The model under review builds one solid part; all positions refer to its coordinate system, in mm. A direction names the side the tool comes from. Round coordinates to 2 decimals unless told otherwise and drop trailing zeros. Loops run counter-clockwise (first coordinate to the right, second up) from the corner with the lowest first, then second, coordinate; pieces in that order, holes last. Notation, with made-up numbers: (-38.5, 59) -> (6.5, 59) arc R20 cw to (6.5, 67) -> close; hole circle Ø9 at (78, -21). An arc over 180 degrees is marked (long way). Use a Markdown table: item, result. Add a question column.
1) Consider section B-B on y = 21.5. Give the boundary of the cut face in (x, z).
2) Consider section C-C on x = -10.5. Give the boundary of the cut face in (y, z).
3) For faces 1 (the flat face through (53.4, 3, -40.1)), 2 (the flat face through (-32.5, 23, -55)), 3 (the flat face through (41, 34, 25)), list the 3-axis set-ups (+Z, -Z, +X, -X, +Y, -Y) from which the entire face can be reached by the end or side of a thin tool; tool diameter is ignored.
4) Consider section D-D on z = -21. Give the boundary of the cut face in (x, y), plus the area to 3 significant figures.
5) Consider section A-A on z = 8.5. State how many separate pieces and enclosed holes the cut face has, plus the area to 3 significant figures.
6) Mouldability with a two-part tool opening along X and no side actions: class faces 4 (the flat face through (38, 38, 53)), 5 (the flat face through (14.5, 5, 2)), 6 (the cylindrical face through (-55.094, 1.479, 32.281)), 7 (the flat face through (-1, 0, -1)) as released by +X, released by -X, zero draft, split by the parting line, or undercut.
7) Insertion check: pin 1 (2.5 mm diameter, centred on x = 18, z = 42, fed in from +Y); pin 2 (2 mm diameter, centred on x = -31, z = 42, fed in from -Y); pin 3 (10 mm diameter, centred on x = 30.5, z = -10.5, fed in from +Y); pin 4 (10 mm diameter, centred on y = 6.5, z = 32, fed in from +X). Each pin has a flat end and moves straight along its axis. Give the tip position at first contact, or say it passes through.
8) Wall thickness on probe 1 along X at (y, z) = (5.4, -16); probe 2 along X at (y, z) = (23.25, 53.5); probe 3 along X at (y, z) = (27, 49): over which ranges is each line inside the solid? List them lowest first.
from build123d import *

# Parameters (mm, degrees)
SKETCH_1_W               = 85
SKETCH_1_H               = 120
EXTRUDE_1_DEPTH          = 40
SKETCH_2_W               = 79
SKETCH_2_H               = 114
CUT_EXTRUDE_1_DEPTH      = 32
SKETCH_3_W               = 42
SKETCH_3_H               = 84
CUT_EXTRUDE_2_DEPTH      = 5
SKETCH_4_W               = 7
SKETCH_4_H               = 7
EXTRUDE_2_DEPTH          = 1.5
SKETCH_5_R               = 1.1
CUT_EXTRUDE_3_DEPTH      = 6
EXTRUDE_3_DEPTH          = 30
SKETCH_7_R               = 1.1
CUT_EXTRUDE_4_DEPTH      = 25
EXTRUDE_4_DEPTH          = 3
SKETCH_9_R               = 1.75
CUT_EXTRUDE_5_DEPTH      = 91.968401107
PATTERN_LINEAR_1_COUNT   = 2
PATTERN_LINEAR_1_PITCH   = 80
MIRROR_1_COPY_1_DEPTH    = 3
MIRROR_1_COPY_2_SKETCH_R = 1.75
MIRROR_1_COPY_2_DEPTH    = 91.968401107
CHAMFER_2_SIZE           = 2
SKETCH_10_W              = 10.9
SKETCH_10_H              = 16.45
CUT_EXTRUDE_6_DEPTH      = 5
SKETCH_11_W              = 13
SKETCH_11_H              = 2
CUT_EXTRUDE_7_DEPTH      = 15.5
SKETCH_12_W              = 40
SKETCH_12_H              = 4
CUT_EXTRUDE_8_DEPTH      = 10
SKETCH_13_W              = 30
SKETCH_13_H              = 4
CUT_EXTRUDE_9_DEPTH      = 5
SKETCH_14_W              = 11
SKETCH_14_H              = 40
CUT_EXTRUDE_10_DEPTH     = 5


with BuildPart() as part:
    # Эскиз1 → Бобышка-Вытянуть1 (new body)
    with BuildSketch(Plane(origin=(0, 0, 0), x_dir=(1, 0, 0), z_dir=(0, 1, 0))):
        Rectangle(SKETCH_1_W, SKETCH_1_H)
    extrude(amount=EXTRUDE_1_DEPTH)

    # Эскиз2 → Вырез-Вытянуть1 (cut)
    with BuildSketch(Plane(origin=(0, 40, 0), x_dir=(1, 0, 0), z_dir=(0, 1, 0))):
        Rectangle(SKETCH_2_W, SKETCH_2_H)
    extrude(amount=-CUT_EXTRUDE_1_DEPTH, mode=Mode.SUBTRACT)

    # Эскиз3 → Вырез-Вытянуть2 (cut)
    with BuildSketch(Plane(origin=(0, 8, 0), x_dir=(1, 0, 0), z_dir=(0, 1, 0))):
        with Locations((-6.5, 0)):
            Rectangle(SKETCH_3_W, SKETCH_3_H)
    extrude(amount=-CUT_EXTRUDE_2_DEPTH, mode=Mode.SUBTRACT)

    # Эскиз4 → Бобышка-Вытянуть2 (add)
    with BuildSketch(Plane(origin=(0, 8, 0), x_dir=(1, 0, 0), z_dir=(0, 1, 0))):
        with Locations((-31, 16)):
            Rectangle(SKETCH_4_W, SKETCH_4_H)
        with Locations((18, 16)):
            Rectangle(SKETCH_4_W, SKETCH_4_H)
        with Locations((-31, -42)):
            Rectangle(SKETCH_4_W, SKETCH_4_H)
        with Locations((18, -42)):
            Rectangle(SKETCH_4_W, SKETCH_4_H)
    extrude(amount=EXTRUDE_2_DEPTH)

    # Эскиз5 → Вырез-Вытянуть3 (cut)
    with BuildSketch(Plane(origin=(0, 9.5, 0), x_dir=(1, 0, 0), z_dir=(0, 1, 0))):
        with Locations(Location((-31, 16, 0), (0, 0, 270))):
            Circle(SKETCH_5_R)
        with Locations(Location((18, 16, 0), (0, 0, 270))):
            Circle(SKETCH_5_R)
        with Locations(Location((18, -42, 0), (0, 0, 270))):
            Circle(SKETCH_5_R)
        with Locations(Location((-31, -42, 0), (0, 0, 270))):
            Circle(SKETCH_5_R)
    extrude(amount=-CUT_EXTRUDE_3_DEPTH, mode=Mode.SUBTRACT)

    # Эскиз6 → Бобышка-Вытянуть3 (add)
    with BuildSketch(Plane(origin=(0, 8, 0), x_dir=(1, 0, 0), z_dir=(0, 1, 0))):
        Polygon((-32.5, 52), (-34.5, 50), (-39.5, 50), (-39.5, 57), (-32.5, 57), align=None)
        Polygon((34.5, 50), (32.5, 52), (32.5, 57), (39.5, 57), (39.5, 50), align=None)
        Polygon((-39.5, -57), (-32.5, -57), (-32.5, -52), (-34.5, -50), (-39.5, -50), align=None)
        Polygon((39.5, -57), (32.5, -57), (32.5, -52), (34.5, -50), (39.5, -50), align=None)
    extrude(amount=EXTRUDE_3_DEPTH)

    # Эскиз7 → Вырез-Вытянуть4 (cut)
    with BuildSketch(Plane(origin=(0, 38, 0), x_dir=(1, 0, 0), z_dir=(0, 1, 0))):
        with Locations(Location((-36, 53.5, 0), (0, 0, 270))):
            Circle(SKETCH_7_R)
        with Locations(Location((36, 53.5, 0), (0, 0, 270))):
            Circle(SKETCH_7_R)
        with Locations(Location((-36, -53.5, 0), (0, 0, 270))):
            Circle(SKETCH_7_R)
        with Locations(Location((36, -53.5, 0), (0, 0, 270))):
            Circle(SKETCH_7_R)
    extrude(amount=-CUT_EXTRUDE_4_DEPTH, mode=Mode.SUBTRACT)

    # Эскиз8 → Бобышка-Вытянуть4 (add)
    with BuildSketch(Plane(origin=(0, 0, 0), x_dir=(1, 0, 0), z_dir=(0, 1, 0))):
        with BuildLine():
            Line((-40.5, 50), (-49.5, 50))
            ThreePointArc((-49.5, 50), (-55.156854249, 47.656854249), (-57.5, 42))
            Line((-57.5, 42), (-57.5, 38))
            ThreePointArc((-57.5, 38), (-55.156854249, 32.343145751), (-49.5, 30))
            Line((-49.5, 30), (-40.5, 30))
            Line((-40.5, 30), (-40.5, 50))
        make_face()
    extrude_4 = extrude(amount=EXTRUDE_4_DEPTH)

    # Эскиз9 → Вырез-Вытянуть5 (cut, through all)
    with BuildSketch(Plane(origin=(0, 3, 0), x_dir=(1, 0, 0), z_dir=(0, 1, 0))):
        with Locations(Location((-49.5, 40, 0), (0, 0, 270))):
            Circle(SKETCH_9_R)
    cut_extrude_5 = extrude(amount=-CUT_EXTRUDE_5_DEPTH, mode=Mode.SUBTRACT)

    # Линейный массив1: Бобышка-Вытянуть4, Вырез-Вытянуть5 ×2
    with Locations(*[(0, 0, i * PATTERN_LINEAR_1_PITCH) for i in range(1, PATTERN_LINEAR_1_COUNT)]):
        add(extrude_4)
        add(cut_extrude_5, mode=Mode.SUBTRACT)

    # Зеркальное отражение1: Бобышка-Вытянуть4, Вырез-Вытянуть5 across plane
    add(extrude_4.mirror(Plane(origin=(0, 0, 0), x_dir=(0, 0, 1), z_dir=(1, 0, 0))))
    add(cut_extrude_5.mirror(Plane(origin=(0, 0, 0), x_dir=(0, 0, 1), z_dir=(1, 0, 0))), mode=Mode.SUBTRACT)

    # Зеркальное отражение1 copy 1 sketch → Зеркальное отражение1 copy 1 (add)
    with BuildSketch(Plane(origin=(0, 0, 80), x_dir=(-1, 0, 0), z_dir=(0, 1, 0))):
        with BuildLine():
            Line((-40.5, -50), (-49.5, -50))
            ThreePointArc((-49.5, -50), (-55.156854249, -47.656854249), (-57.5, -42))
            Line((-57.5, -42), (-57.5, -38))
            ThreePointArc((-57.5, -38), (-55.156854249, -32.343145751), (-49.5, -30))
            Line((-49.5, -30), (-40.5, -30))
            Line((-40.5, -30), (-40.5, -50))
        make_face()
    extrude(amount=MIRROR_1_COPY_1_DEPTH)

    # Зеркальное отражение1 copy 2 sketch → Зеркальное отражение1 copy 2 (cut, through all)
    with BuildSketch(Plane(origin=(0, 3, 80), x_dir=(-1, 0, 0), z_dir=(0, 1, 0))):
        with Locations((-49.5, -40)):
            Circle(MIRROR_1_COPY_2_SKETCH_R)
    extrude(amount=-MIRROR_1_COPY_2_DEPTH, mode=Mode.SUBTRACT)

    # Фаска2
    chamfer_2_edges = [part.edges().sort_by_distance(p)[0] for p in [
        (-49.5, 3, -41.75),
        (-49.5, 3, 38.25),
        (49.5, 3, -41.75),
        (51.25, 3, 40),
    ]]
    chamfer(chamfer_2_edges, length=CHAMFER_2_SIZE)

    # Эскиз10 → Вырез-Вытянуть6 (cut)
    with BuildSketch(Plane.XY.offset(60)):
        with Locations((-23.05, 33.775)):
            Rectangle(SKETCH_10_W, SKETCH_10_H)
    extrude(amount=-CUT_EXTRUDE_6_DEPTH, mode=Mode.SUBTRACT)

    # Эскиз11 → Вырез-Вытянуть7 (cut)
    with BuildSketch(Plane(origin=(0, 40, 0), x_dir=(1, 0, 0), z_dir=(0, 1, 0))):
        with Locations((-23.05, -57)):
            Rectangle(SKETCH_11_W, SKETCH_11_H)
    extrude(amount=-CUT_EXTRUDE_7_DEPTH, mode=Mode.SUBTRACT)

    # Эскиз12 → Вырез-Вытянуть8 (cut)
    with BuildSketch(Plane(origin=(42.5, 0, 0), x_dir=(0, 0, -1), z_dir=(1, 0, 0))):
        with Locations((-5, 34)):
            Rectangle(SKETCH_12_W, SKETCH_12_H)
        with Locations((-5, 26)):
            Rectangle(SKETCH_12_W, SKETCH_12_H)
        with Locations((-5, 18)):
            Rectangle(SKETCH_12_W, SKETCH_12_H)
        with Locations((-5, 10)):
            Rectangle(SKETCH_12_W, SKETCH_12_H)
    extrude(amount=-CUT_EXTRUDE_8_DEPTH, mode=Mode.SUBTRACT)

    # Эскиз13 → Вырез-Вытянуть9 (cut)
    with BuildSketch(Plane.ZY.offset(42.5)):
        with Locations((-25, 34)):
            Rectangle(SKETCH_13_W, SKETCH_13_H)
        with Locations((-25, 26)):
            Rectangle(SKETCH_13_W, SKETCH_13_H)
        with Locations((-25, 18)):
            Rectangle(SKETCH_13_W, SKETCH_13_H)
        with Locations((-25, 10)):
            Rectangle(SKETCH_13_W, SKETCH_13_H)
    extrude(amount=-CUT_EXTRUDE_9_DEPTH, mode=Mode.SUBTRACT)

    # Эскиз14 → Вырез-Вытянуть10 (cut)
    with BuildSketch(Plane(origin=(0, 8, 0), x_dir=(1, 0, 0), z_dir=(0, 1, 0))):
        with Locations((34, -5)):
            Rectangle(SKETCH_14_W, SKETCH_14_H)
    extrude(amount=-CUT_EXTRUDE_10_DEPTH, mode=Mode.SUBTRACT)


solid = part.part
Result set:
| question | item | result |
|---|---|---|
| 1 | outline | (-42.5, -60) -> (42.5, -60) -> (42.5, 60) -> (-42.5, 60) -> close; hole (-39.5, -50) -> (-34.5, -50) -> (-32.5, -52) -> (-32.5, -57) -> (32.5, -57) -> (32.5, -52) -> (34.5, -50) -> (39.5, -50) -> (39.5, 50) -> (34.5, 50) -> (32.5, 52) -> (32.5, 57) -> (-32.5, 57) -> (-32.5, 52) -> (-34.5, 50) -> (-39.5, 50) -> close; hole circle Ø2.2 at (-36, -53.5); hole circle Ø2.2 at (-36, 53.5); hole circle Ø2.2 at (36, -53.5); hole circle Ø2.2 at (36, 53.5) |
| 2 | outline | (0, -60) -> (40, -60) -> (40, -57) -> (8, -57) -> (8, -42) -> (3, -42) -> (3, 42) -> (8, 42) -> (8, 57) -> (40, 57) -> (40, 60) -> (0, 60) -> close |
| 3 | face 1 | +Z, -Z, +X, +Y |
| 3 | face 2 | +Y |
| 3 | face 3 | +X |
| 4 | outline | (-42.5, 0) -> (42.5, 0) -> (42.5, 40) -> (39.5, 40) -> (39.5, 8) -> (14.5, 8) -> (14.5, 3) -> (-27.5, 3) -> (-27.5, 8) -> (-42.5, 8) -> close; (-42.5, 12) -> (-39.5, 12) -> (-39.5, 16) -> (-42.5, 16) -> close; (-42.5, 20) -> (-39.5, 20) -> (-39.5, 24) -> (-42.5, 24) -> close; (-42.5, 28) -> (-39.5, 28) -> (-39.5, 32) -> (-42.5, 32) -> close; (-42.5, 36) -> (-39.5, 36) -> (-39.5, 40) -> (-42.5, 40) -> close |
| 4 | area | 614 mm2 |
| 5 | separate pieces | 5 |
| 5 | enclosed holes | 0 |
| 5 | area | 559 mm2 |
| 6 | face 4 | undercut |
| 6 | face 5 | undercut |
| 6 | face 6 | released by -X |
| 6 | face 7 | zero draft |
| 7 | pin 1 | y = 9.5 |
| 7 | pin 2 | y = 0 |
| 7 | pin 3 | y = 8 |
| 7 | pin 4 | x = 57.12 |
| 8 | probe 1 | -42.5 to -32.1, -29.9 to -27.5, 14.5 to 16.9, 19.1 to 42.5 |
| 8 | probe 2 | -42.5 to -37.1, -34.9 to -32.5, 32.5 to 34.9, 37.1 to 42.5 |
| 8 | probe 3 | -42.5 to -39.5, 39.5 to 42.5 |
